Read the model definition and answer for the solid it produces. Units are mm, in the model's axes. A direction names the side the tool comes from. Coordinates: 2 decimals unless noted, no trailing zeros. Loops run counter-clockwise (first coordinate to the right, second up) from the corner with the lowest first, then second, coordinate; pieces in that order, holes last. Notation, with made-up numbers: (2.5, -24.75) -> (38.5, -24.75) arc R12 ccw to (38.5, -7.75) -> close; hole circle Ø10 at (63.25, -34.5). An arc over 180 degrees is marked (long way). Answer as a JSON object with one key per item and string values. Group by question number.
Q1. The part is cut by section A-A on y = 1.3. Write down the section's boundary in (x, z), and give its area (3 significant figures).
Q2. For faces 5 (the flat face through (0, 3.7, -1.3)), 6 (the flat face through (12, 3.5, -3)), 7 (the flat face through (7, 3.9, 3)), determine the directions among +Z, -Z, +X, -X, +Y, -Y from which every point of the face is accessible in a straight line to the end or side of a thin tool.
Q3. The part is cut by section B-B on y = 2.85. Write down the section's boundary in (x, z), and give its area (3 significant figures).
Q4. Determine the mould class of faces 1 (the flat face through (7.6, -0.2, -4.5)), 2 (the flat face through (10.6, 2, -3)), 3 (the flat face through (9.3, 0, -3)), 4 (the flat face through (11, 2, -3)) for opening direction X: released by +X, released by -X, zero draft, split by the parting line, or undercut.
Q5. Straight lines are drawn through the part: line 1 along Y through (x, z) = (-0.25, -4.5); line 2 along X through (y, z) = (1.3, -3.5); line 3 along Y through (x, z) = (2.5, -2.25). For each, find the intervals that lie inside material, in ascending order. Write a range as [from, to].
Q6. Each of these flat-tipped pins is pushed along its axis until it touches: P1, Ø2, axis at x = 8, y = 2, coming from the -Z side; P2, Ø1.5, axis at x = 6, y = 1, coming from the +Z side; P3, Ø2, axis at x = -3, y = 3, coming from the -Z side. Where does it stop, or does it pass through?
Autodesk Inventor part; units mm, degrees
ref_plane "YZ Plane" through (0, 0, 0) normal (1, 0, 0) x (0, 1, 0)
ref_plane "XZ Plane" through (0, 0, 0) normal (0, 1, 0) x (-1, 0, 0)
ref_plane "XY Plane" through (0, 0, 0) normal (0, 0, 1) x (1, 0, 0)
sketch "Sketch1" plane through (0, 0, 0) normal (0, 1, 0) x (-1, 0, 0)
  circle A0 centre (0, 0) radius 10.01
  dimension "d0" = 20.02
extrude "Extrusion1" add sketch "Sketch1" along normal blind 3.5
fillet "Fillet1" radius 1 1 edges at (10.01, 3.5, 0)
fillet "Fillet2" radius 1 1 edges at (10.01, 0, 0)
sketch "Sketch2" plane through (0, 3.5, 0) normal (0, 1, 0) x (1, 0, 0)
  line L0 (0, 0) -> (0, -1.5)
  line L1 (0, -1.5) -> (14, -1.5)
  line L2 (14, -1.5) -> (14, -4.5)
  line L3 (14, -4.5) -> (0, -4.5)
  line L4 (0, -4.5) -> (0, -1.5)
  dimension "d5" = 1.5
  dimension "d6" = 14
  dimension "d7" = 3
extrude "Extrusion2" add sketch "Sketch2" along normal blind 0.4
sketch "Sketch3" plane through (0, 0, 0) normal (0, -1, 0) x (1, 0, 0)
  line L0 (0, 0) -> (0, -1.5)
  line L1 (0, -1.5) -> (11, -1.5)
  line L2 (11, -1.5) -> (11, -4.5)
  line L3 (11, -4.5) -> (0, -4.5)
  line L4 (0, -4.5) -> (0, -1.5)
  dimension "d10" = 1.5
  dimension "d11" = 11
  dimension "d12" = 3
extrude "Extrusion3" add sketch "Sketch3" along normal blind 0.4
sketch "Sketch4" plane through (0, 0, 0) normal (0, 1, 0) x (1, 0, 0)
  line L0 (11, 4.5) -> (11, 1.5)
  line L1 (11, 1.5) -> (11, 4.5)
  line L2 (11, 4.5) -> (10.6, 4.5)
  line L3 (10.6, 4.5) -> (10.6, 1.5)
  line L4 (10.6, 1.5) -> (11, 1.5)
  point P0 (0, 0)
  dimension "d15" = 0.4
extrude "Extrusion4" add sketch "Sketch4" along normal blind 3.5
fillet "Fillet3" radius 0.4 1 edges at (11, -0.4, -3)
fillet "Fillet4" radius 0.4 1 edges at (10.6, 0, -3)
sketch "Sketch5" plane through (0, 3.5, 0) normal (0, 1, 0) x (1, 0, 0)
  line L0 (10.6, 4.5) -> (10.6, 1.5)
  line L1 (10.6, 1.5) -> (14, 1.5)
  line L2 (14, 1.5) -> (14, 4.5)
  line L3 (14, 4.5) -> (10.6, 4.5)
  line L4 (10.6, 4.5) -> (10.6, 1.5)
  point P0 (0, 0)
  dimension "d20" = 3
  dimension "d21" = 3.4
extrude "Extrusion5" add sketch "Sketch5" along normal blind 0.4
sketch "Sketch6" plane through (0, 3.5, 0) normal (0, 1, 0) x (1, 0, 0)
  line L0 (-1.4984, 2.512) -> (1.5521, 2.512) construction
  line L1 (1.5521, 2.512) -> (1.5521, 0.1186) construction
  line L2 (1.5521, 0.1186) -> (-1.4984, 0.1186) construction
  line L3 (-1.4984, 0.1186) -> (-1.4984, 2.512) construction
  line L4 (1.231, 1.1511) -> (0.1985, 1.1511)
  line L5 (0.1985, 1.1511) -> (0.1985, 0.1186)
  line L6 (0.1985, 0.1186) -> (-0.1424, 0.1186)
  line L7 (-0.1424, 0.1186) -> (-0.1424, 1.1511)
  line L8 (-0.1424, 1.1511) -> (-1.1748, 1.1511)
  line L9 (-1.1748, 1.1511) -> (-1.1748, 1.4796)
  line L10 (-1.1748, 1.4796) -> (-0.1424, 1.4796)
  line L11 (-0.1424, 1.4796) -> (-0.1424, 2.512)
  line L12 (-0.1424, 2.512) -> (0.1985, 2.512)
  line L13 (0.1985, 2.512) -> (0.1985, 1.4796)
  line L14 (0.1985, 1.4796) -> (1.231, 1.4796)
  line L15 (1.231, 1.4796) -> (1.231, 1.1511)
  point P0 (0, 0)
extrude "Extrusion6" add sketch "Sketch6" along normal mid plane 0.4
properties part number "RJD2032C1ST1"
Final values:
{
 "1": {"outline": "circle Ø20.02 at (0, 0); (10.6, -4.5) -> (11, -4.5) -> (11, -1.5) -> (10.6, -1.5) -> close", "area": "316 mm2"},
 "2": {"face 5": "-Z, -X, +Y", "face 6": "+Z, -Z, +X, -Y", "face 7": "+Z, -Z, +X, -X, +Y"},
 "3": {"outline": "circle Ø19.89 at (0, 0); (10.6, -4.5) -> (11, -4.5) -> (11, -1.5) -> (10.6, -1.5) -> close", "area": "312 mm2"},
 "4": {"face 1": "zero draft", "face 2": "undercut", "face 3": "undercut", "face 4": "released by +X"},
 "5": {"line 1": "y = [0, 3.5]", "line 2": "x = [-9.38, 9.38], [10.6, 11]", "line 3": "y = [-0.4, 3.5]"},
 "6": {"P1": "stops at z = -7.16", "P2": "stops at z = 8.52", "P3": "stops at z = -9.79"}
}
